Design review of the part shown in the three views and the two pictorial views. Dimensions are in mm from the part's minimum x, y and z. Coordinates: 2 decimals unless noted, no trailing zeros.
Q1. For L1, parallel to Z at x = 72, y = 0.85; L2, parallel to Z at x = 16, y = 1.25; L3, parallel to Z at x = 8.5, y = 0.65, list the stretches that pass through material, from the lowest coordinate up.
Q2. Take a section at A-A, the plane z = 29.5. State how many separate pieces and enclosed holes the cut face has.
Q3. For pin 1 Ø12 at (x, z) = (64.5, 6) entering from -Y, flat-tipped, find the tip position at first contact; note if it passes through.
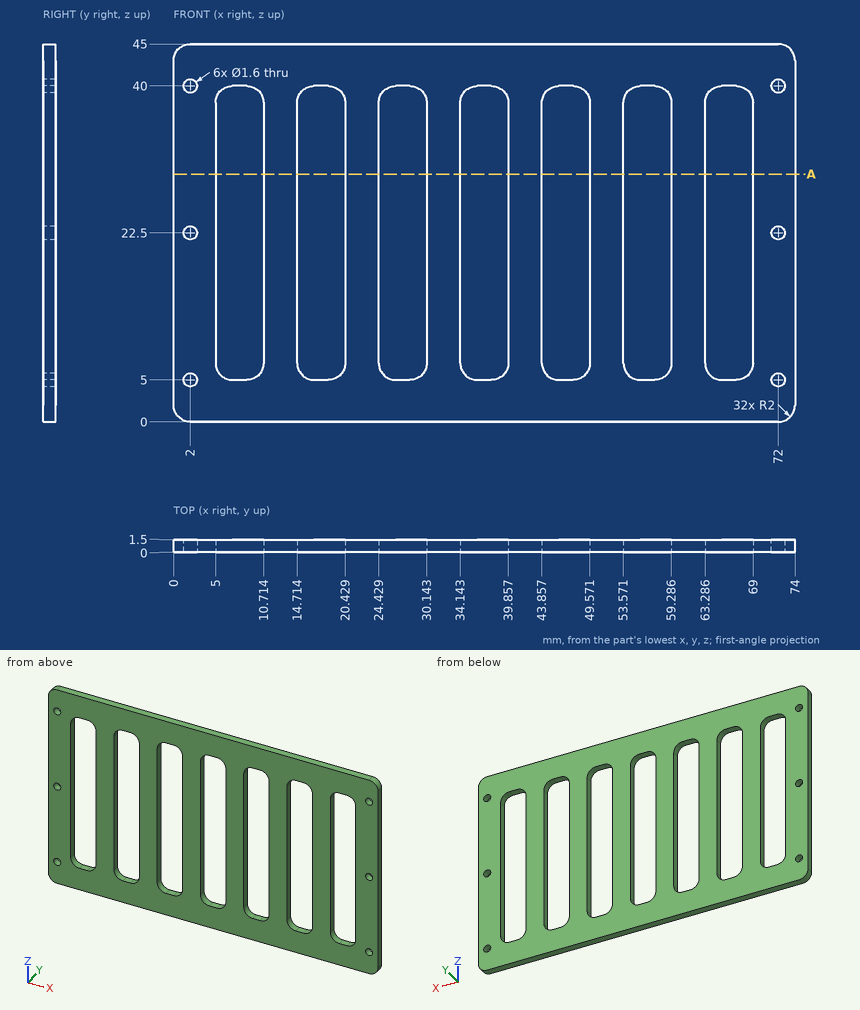
Responses:
1. L1: z = 0 to 4.2, 5.8 to 21.7, 23.3 to 39.2, 40.8 to 45
1. L2: z = 0 to 5.13, 39.87 to 45
1. L3: z = 0 to 5, 40 to 45
2. separate pieces: 8
2. enclosed holes: 0
3. pin 1: stops at y = 0
